```python
from build123d import *

# Parameters (mm, degrees)
SKETCH_1_R      = 15
SKETCH_1_R_2    = 1.75
EXTRUDE_1_DEPTH = 14
FILLET_1_R      = 2
FILLET_2_R      = 7


with BuildPart() as part:
    # Эскиз1 → Бобышка-Вытянуть1 (new body)
    with BuildSketch(Plane.XY):
        Circle(SKETCH_1_R)
        Circle(SKETCH_1_R_2, mode=Mode.SUBTRACT)
    extrude(amount=EXTRUDE_1_DEPTH)

    # Скругление1
    fillet_1_edges = [part.edges().sort_by_distance(p)[0] for p in [
        (-15, 0, 14),
    ]]
    fillet(fillet_1_edges, radius=FILLET_1_R)

    # Скругление2
    fillet_2_edges = [part.edges().sort_by_distance(p)[0] for p in [
        (-15, 0, 0),
    ]]
    fillet(fillet_2_edges, radius=FILLET_2_R)


solid = part.part
```
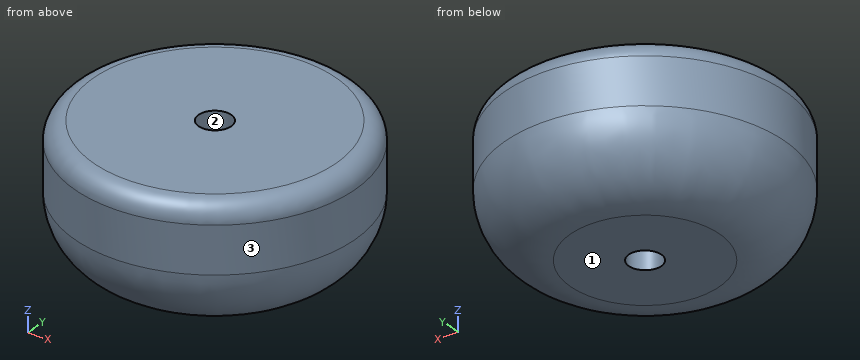
The listing builds one solid part. Answer for the finished solid, in the listing's coordinates (mm). Face numbers are marked on the shaded views. Round coordinates to 2 decimals unless told otherwise and drop trailing zeros. Write each loop counter-clockwise with the first axis right and the second up, starting at its lowest first coordinate (ties: lowest second). Pieces come first, ordered by that corner, then holes. Notation, with made-up numbers: (76, 38) -> (116, 38) arc R20 ccw to (116, 44) -> close; hole circle Ø10 at (86.25, 82.5). An arc over 180 degrees is marked (long way). Answer as a JSON object with one key per item and string values. Group by question number.
Q1. Straight lines are drawn through the part: line 1 along Y through (x, z) = (0, 8); line 2 along Y through (x, z) = (-7.5, 7); line 3 along Y through (x, z) = (-1, 10.25). For each, find the intervals that lie inside material, in ascending order.
Q2. Section C-C (z = 11.25) is taken. Write down the section's boundary in (x, y), plus the area to 3 significant figures.
Q3. Section A-A (x = 0) is taken. Write down the section's boundary in (y, z), plus the area to 3 significant figures.
Q4. Determine the mould class of the marked faces 1, 2 and 3 for opening direction X: pulls with the +X half, pulls with the -X half, needs draft (parallel to the pull), parting line crosses it, or undercut.
Q5. Each of these flat-tipped pins is pushed along its axis until it touches: pin 1 Ø2 at (x, y) = (-11, 9) entering from +Z; pin 2 Ø3 at (x, y) = (9.5, 3.5) entering from -Z; pin 3 Ø2 at (y, z) = (6, 7) entering from -X. Where does it stop, or does it pass through?
Check values:
{
 "1": {"line 1": "-15 to -1.75, 1.75 to 15", "line 2": "-12.99 to 12.99", "line 3": "-14.97 to -1.44, 1.44 to 14.97"},
 "2": {"outline": "circle Ø30 at (0, 0); hole circle Ø3.5 at (0, 0)", "area": "697 mm^2"},
 "3": {"outline": "(-15, 7) arc R7 ccw to (-8, 0) -> (-1.75, 0) -> (-1.75, 14) -> (-13, 14) arc R2 ccw to (-15, 12) -> close; (1.75, 0) -> (8, 0) arc R7 ccw to (15, 7) -> (15, 12) arc R2 ccw to (13, 14) -> (1.75, 14) -> close", "area": "348 mm^2"},
 "4": {"face 1": "needs draft", "face 2": "undercut", "face 3": "parting line crosses it"},
 "5": {"pin 1": "z = 13.99", "pin 2": "z = 0.03", "pin 3": "x = -14.14"}
}
